```python
from build123d import *

# Parameters (mm, degrees)
CROQUIS1_W              = 50.8
CROQUIS1_H              = 25.4
CROQUIS1_W_2            = 47.8
CROQUIS1_H_2            = 22.4
SALIENTE_EXTRUIR1_DEPTH = 440
CORTAR_EXTRUIR1_DEPTH   = 26


with BuildPart() as part:
    # Croquis1 → Saliente-Extruir1 (new body)
    with BuildSketch(Plane.XY):
        Rectangle(CROQUIS1_W, CROQUIS1_H)
        Rectangle(CROQUIS1_W_2, CROQUIS1_H_2, mode=Mode.SUBTRACT)
    extrude(amount=SALIENTE_EXTRUIR1_DEPTH)

    # Croquis2 → Cortar-Extruir1 (cut)
    with BuildSketch(Plane(origin=(0, 12.7, 0), x_dir=(1, 0, 0), z_dir=(0, 1, 0))):
        Polygon((-25.4, 0), (25.4, -50.8), (25.4, 0), align=None)
        Polygon((25.4, -389.2), (25.4, -440), (-25.4, -440), align=None)
    extrude(amount=-CORTAR_EXTRUIR1_DEPTH, mode=Mode.SUBTRACT)


solid = part.part
```
For this review, take the finished solid that the model builds, in its own axes (mm). A direction names the side the tool comes from. Give positions to 0.01 mm unless a question says otherwise; leave off trailing zeros. Write each loop counter-clockwise with the first axis right and the second up, starting at its lowest first coordinate (ties: lowest second). Pieces come first, ordered by that corner, then holes.
Item 1: The part is to be moulded in two halves that separate along Y. For faces 1 (the face through (0, 12.7, 217)), 2 (the face through (-25.4, 0, 217)), 3 (the face through (0, -11.2, 217)), 4 (the face through (0, -12.7, 217)), say which applies: +Y half, -Y half, draft (parallel to the pull), parting line (faces both ways), or undercut.
Item 2: Take a section at C-C (y = -2.75). Give the boundary of the cut face in (x, z).
Item 3: Take a section at B-B (z = 106.5). Give the boundary of the cut face in (x, y).
Item 4: Wall thickness on probe 1 along Y at (x, z) = (-12.5, 67); probe 2 along X at (y, z) = (-6, 247); probe 3 along X at (y, z) = (3, 400): over which ranges is each line inside the solid? List them lowest first.
Item 5: Machinability: for faces 5 (the face through (23.9, 0, 218)), 6 (the face through (25.4, 0, 218)), which of the approach directions +Z, -Z, +X, -X, +Y, -Y give a long, thin tool a straight path to every point of the face, cutting with its end or side? Answer none if there is none.
Item 6: Take a section at A-A (x = -14.5). Give the boundary of the cut face in (y, z).
Established:
1. face 1: +Y half
1. face 2: draft
1. face 3: undercut
1. face 4: -Y half
2. outline: (-25.4, 0) - (-23.9, 1.5) - (-23.9, 438.5) - (-25.4, 440) - close; (23.9, 49.3) - (25.4, 50.8) - (25.4, 389.2) - (23.9, 390.7) - close
3. outline: (-25.4, -12.7) - (25.4, -12.7) - (25.4, 12.7) - (-25.4, 12.7) - close; hole (-23.9, -11.2) - (23.9, -11.2) - (23.9, 11.2) - (-23.9, 11.2) - close
4. probe 1: y = -12.7 to -11.2, 11.2 to 12.7
4. probe 2: x = -25.4 to -23.9, 23.9 to 25.4
4. probe 3: x = -25.4 to -23.9
5. face 5: +Z, -Z
5. face 6: +Z, -Z, +X, +Y, -Y
6. outline: (-12.7, 10.9) - (-11.2, 10.9) - (-11.2, 429.1) - (-12.7, 429.1) - close; (11.2, 10.9) - (12.7, 10.9) - (12.7, 429.1) - (11.2, 429.1) - close
